from build123d import *

# Parameters (mm, degrees)
SKETCH1_W           = 10
SKETCH1_H           = 5
BOSS_EXTRUDE2_DEPTH = 50
SKETCH2_R           = 1.5
CUT_EXTRUDE1_DEPTH  = 100
SKETCH5_R           = 2
CUT_EXTRUDE3_DEPTH  = 100
SKETCH6_W           = 50
SKETCH6_H           = 15
BOSS_EXTRUDE3_DEPTH = 3


with BuildPart() as part:
    # Sketch1 → Boss-Extrude2 (new, symmetric)
    with BuildSketch(Plane.XY):
        with BuildLine():
            ThreePointArc((-20, 0), (0, -20), (20, 0))
            Line((20, 0), (25, 0))
            Line((25, 0), (25, -21))
            Line((25, -21), (-25, -21))
            Line((-25, -21), (-25, 0))
            Line((-25, 0), (-20, 0))
        make_face()
        with Locations((-30, -18.5)):
            Rectangle(SKETCH1_W, SKETCH1_H)
        with Locations((30, -18.5)):
            Rectangle(SKETCH1_W, SKETCH1_H)
    extrude(amount=BOSS_EXTRUDE2_DEPTH, both=True)

    # Sketch2 → Cut-Extrude1 (cut)
    with BuildSketch(Plane(origin=(0, -16, 0), x_dir=(1, 0, 0), z_dir=(0, 1, 0))):
        with Locations(Location((-30, 40, 0), (0, 0, 270))):
            Circle(SKETCH2_R)
        with Locations(Location((-30, 0, 0), (0, 0, 270))):
            Circle(SKETCH2_R)
        with Locations(Location((-30, -40, 0), (0, 0, 270))):
            Circle(SKETCH2_R)
        with Locations(Location((30, 40, 0), (0, 0, 270))):
            Circle(SKETCH2_R)
        with Locations(Location((30, 0, 0), (0, 0, 270))):
            Circle(SKETCH2_R)
        with Locations(Location((30, -40, 0), (0, 0, 270))):
            Circle(SKETCH2_R)
    extrude(amount=-CUT_EXTRUDE1_DEPTH, mode=Mode.SUBTRACT)

    # Sketch5 → Cut-Extrude3 (cut)
    with BuildSketch(Plane(origin=(25, 0, 0), x_dir=(0, 0, -1), z_dir=(1, 0, 0))):
        with Locations((-40, -5)):
            Circle(SKETCH5_R)
        with Locations((0, -5)):
            Circle(SKETCH5_R)
        with Locations((40, -5)):
            Circle(SKETCH5_R)
    extrude(amount=-CUT_EXTRUDE3_DEPTH, mode=Mode.SUBTRACT)

    # Sketch6 → Boss-Extrude3 (add)
    with BuildSketch(Plane.XY.offset(50)):
        with Locations((0, -13.5)):
            Rectangle(SKETCH6_W, SKETCH6_H)
    boss_extrude3 = extrude(amount=BOSS_EXTRUDE3_DEPTH)

    # Mirror2: Boss-Extrude3 across plane
    add(boss_extrude3.mirror(Plane.XY))


solid = part.part
Here's how the part is built. I have some questions about the finished solid (model axes, mm). A direction names the side the tool comes from. Round coordinates to 2 decimals unless told otherwise and drop trailing zeros. Loops run counter-clockwise (first coordinate to the right, second up) from the corner with the lowest first, then second, coordinate; pieces in that order, holes last. Notation, with made-up numbers: (85, 80.25) - (117, 80.25) arc R8 ccw to (117, 89.25) - close; hole circle Ø1 at (89.25, 44.25). An arc over 180 degrees is marked (long way). One line per question, with ' | ' between items. Start each with the question number.
Q1. I want a section at B-B (z = -24). Write out the boundary of the cut face in (x, y), then the cut area to 3 significant figures.
Q2. I want a section at D-D (x = 0). Write out the boundary of the cut face in (y, z), then the cut area to 3 significant figures.
Q3. Will these pins go through, and if not, where does the flat tip stop? pin 1 (5 mm diameter, centred on x = -30, z = -40, fed in from +Y); pin 2 (6.5 mm diameter, centred on y = -5, z = 40, fed in from -X); pin 3 (3.5 mm diameter, centred on x = 30, z = -40, fed in from -Y); pin 4 (4.5 mm diameter, centred on x = 21.5, y = -2.5, fed in from -Z).
Q4. For faces 1 (the flat face through (22, -3, -50)), 2 (the cylindrical face through (0, -20, 1)), 3 (the flat face through (22, -3, 50)), which set-ups out of +Z, -Z, +X, -X, +Y, -Y let a thin tool reach every point of the face, with its end or its side?
Q5. We'd pull the mould along Y, two halves only. Please class faces 4 (the cylindrical face through (-22, -7, 0)), 5 (the flat face through (-28, -16, 1)), 6 (the flat face through (0, -11, 50)): +Y half, -Y half, draft (parallel to the pull), parting line (faces both ways), or undercut.
Q6. I want a section at C-C (y = -10.5). Write out the boundary of the cut face in (x, z).
Q7. Please list where these lines run through material, in increasing order: line 1 (Z direction, x = -19.75, y = -5); line 2 (Y direction, x = 22, z = 40); line 3 (Z direction, x = 6, y = -9.75). Write a range as [from, to].
Q8. I want a section at A-A (x = 30). Write out the boundary of the cut face in (y, z).
Response values:
1) outline: (-35, -21) - (35, -21) - (35, -16) - (25, -16) - (25, 0) - (20, 0) arc R20 cw to (-20, 0) - (-25, 0) - (-25, -16) - (-35, -16) - close | area: 522 mm²
2) outline: (-21, -53) - (-6, -53) - (-6, -50) - (-20, -50) - (-20, 50) - (-6, 50) - (-6, 53) - (-21, 53) - close | area: 190 mm²
3) pin 1: stops at y = -16 | pin 2: stops at x = -25 | pin 3: stops at y = -21 | pin 4: stops at z = -50
4) face 1: -Z, +X, -X, +Y | face 2: +Y | face 3: +Z, +X, -X, +Y
5) face 4: undercut | face 5: +Y half | face 6: draft
6) outline: (-25, -53) - (25, -53) - (25, 53) - (-25, 53) - close; hole (-17.02, -50) - (17.02, -50) - (17.02, 50) - (-17.02, 50) - close
7) line 1: z = [-50, -42], [-38, -2], [2, 38], [42, 50] | line 2: y = [-21, -7], [-3, 0] | line 3: z = [-53, -50], [50, 53]
8) outline: (-21, -50) - (-16, -50) - (-16, -41.5) - (-21, -41.5) - close; (-21, -38.5) - (-16, -38.5) - (-16, -1.5) - (-21, -1.5) - close; (-21, 1.5) - (-16, 1.5) - (-16, 38.5) - (-21, 38.5) - close; (-21, 41.5) - (-16, 41.5) - (-16, 50) - (-21, 50) - close
